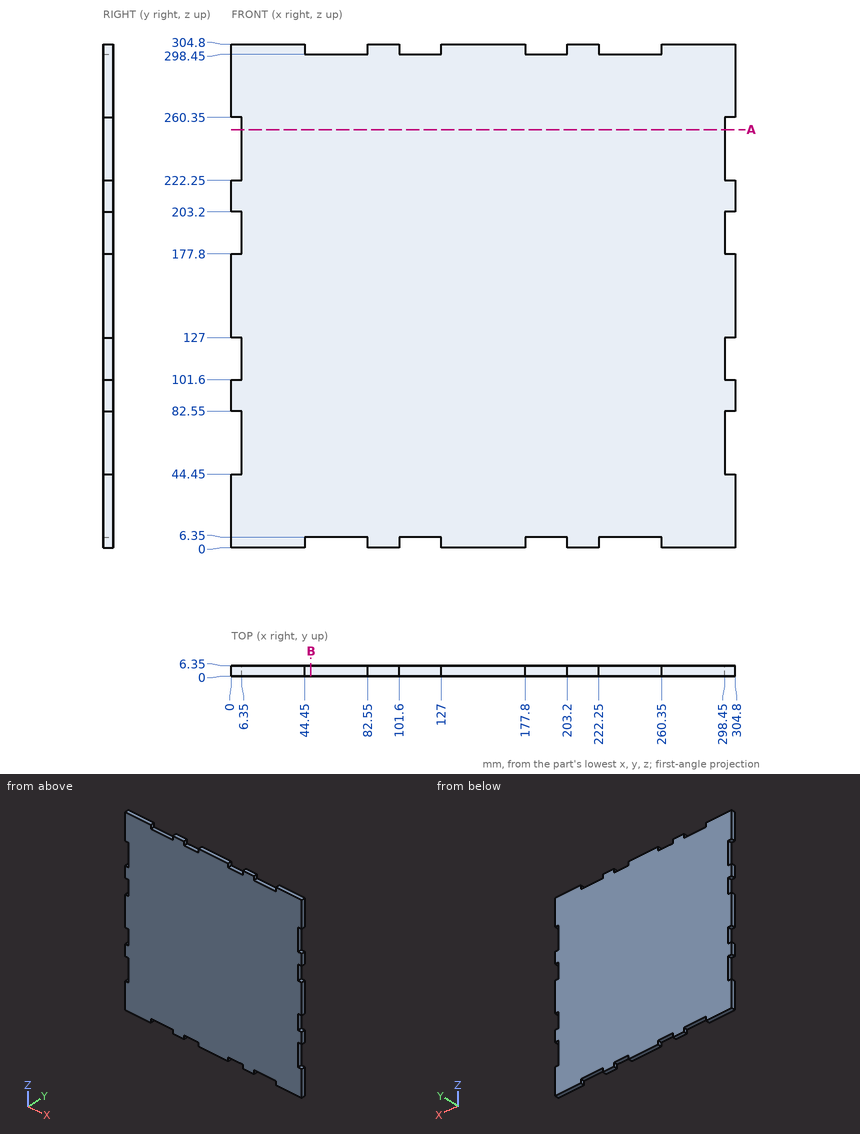
Geometry: see drawing. Coordinates: mm, zero at the bounding-box minimum. Coordinates: 2 decimals unless noted, no trailing zeros. Write each loop counter-clockwise with the first axis right and the second up, starting at its lowest first coordinate (ties: lowest second). Pieces come first, ordered by that corner, then holes. Notation, with made-up numbers: M -17,-21 L 40,-21 A33 ccw 40,18 Z; hole C -9.5,84 d9. An arc over 180 degrees is marked long. Use CSV: the item, a comma, the result in double quotes. Start each with the question number.
1. Cut plane B-B on x = 48. Return the cut outline in (y, z).
2. Ray query, probe 1 along X at (y, z) = (5, 72). Return the intervals inside material, ascending.
3. Cut plane A-A on z = 253. Return the cut outline in (x, y), plus the area to 3 significant figures.
4. First-contact query: P1, Ø1.9, axis at y = 4.5, z = 192, coming from the -X side; P2, Ø3, axis at y = 3.5, z = 111.5, coming from the +X side. Flat tips, straight axial feed; report the tip coordinate or a pass-through.
Entries:
1,outline,"M 0,6.35 L 6.35,6.35 L 6.35,298.45 L 0,298.45 Z"
2,probe 1,"6.35 to 298.45"
3,outline,"M 6.35,0 L 298.45,0 L 298.45,6.35 L 6.35,6.35 Z"
3,area,"1,850 mm²"
4,P1,"x = 6.35"
4,P2,"x = 298.45"
